Input: part model. Units: mm. Frame: model coordinates. Face numbers are marked on the shaded views. Coordinates: 2 decimals unless noted, no trailing zeros. Loops run counter-clockwise (first coordinate to the right, second up) from the corner with the lowest first, then second, coordinate; pieces in that order, holes last. Notation, with made-up numbers: (15, -22) - (21, -22) arc R23 ccw to (21, -2) - close; hole circle Ø4 at (61, 54.25). An arc over 180 degrees is marked (long way). Write item = value, one per line. Start each with the question number.
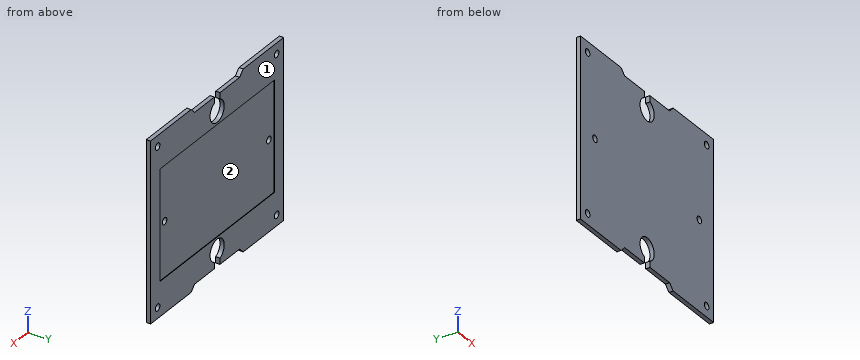
from build123d import *

# Parameters (mm, degrees)
SKETCH1_W              = 94
SKETCH1_H              = 83
SKETCH1_R              = 1.5875
BOSS_EXTRUDE1_DEPTH    = 2
SKETCH2_W              = 81
SKETCH2_H              = 51
CUT_EXTRUDE1_DEPTH     = 0.2
CUT_EXTRUDE2_START     = -2
CUT_EXTRUDE2_OUTLINE_R = 1.6
CUT_EXTRUDE2_DEPTH     = 2


# Read off the part's stored shape, not the designer's step: Cut-Extrude2
with BuildPart() as part:
    # Sketch1 → Boss-Extrude1 (new body)
    with BuildSketch(Plane(origin=(0, 0, 0), x_dir=(1, 0, 0), z_dir=(0, 1, 0))):
        Rectangle(SKETCH1_W, SKETCH1_H)
        with Locations(Location((-42, 36.5, 0), (0, 0, 270))):
            Circle(SKETCH1_R, mode=Mode.SUBTRACT)
        with Locations(Location((42, 36.5, 0), (0, 0, 270))):
            Circle(SKETCH1_R, mode=Mode.SUBTRACT)
        with Locations(Location((42, -36.5, 0), (0, 0, 270))):
            Circle(SKETCH1_R, mode=Mode.SUBTRACT)
        with Locations(Location((-42, -36.5, 0), (0, 0, 270))):
            Circle(SKETCH1_R, mode=Mode.SUBTRACT)
    extrude(amount=BOSS_EXTRUDE1_DEPTH)

    # Sketch2 → Cut-Extrude1 (cut)
    with BuildSketch(Plane(origin=(0, 2, 0), x_dir=(1, 0, 0), z_dir=(0, 1, 0))):
        Rectangle(SKETCH2_W, SKETCH2_H)
    extrude(amount=-CUT_EXTRUDE1_DEPTH, mode=Mode.SUBTRACT)

    # Cut-Extrude2 outline → Cut-Extrude2 (cut)
    with BuildSketch(Plane(origin=(0, 2, 0), x_dir=(1, 0, 0), z_dir=(0, 1, 0)).offset(CUT_EXTRUDE2_START)):
        with Locations((36.83, 0)):
            Circle(CUT_EXTRUDE2_OUTLINE_R)
        with Locations((-36.83, 0)):
            Circle(CUT_EXTRUDE2_OUTLINE_R)
        with BuildLine():
            Line((15.875, -38.96), (2, -38.96))
            Line((2, -38.96), (2, -36.082575695))
            ThreePointArc((2, -36.082575695), (0, -26.5), (-2, -36.082575695))
            Line((-2, -36.082575695), (-2, -38.96))
            Line((-2, -38.96), (-15.875, -38.96))
            Line((-15.875, -38.96), (-18.415, -41.5))
            Line((-18.415, -41.5), (18.415, -41.5))
            Line((18.415, -41.5), (15.875, -38.96))
        make_face()
        with BuildLine():
            Line((2, 36.082575695), (2, 38.96))
            Line((2, 38.96), (15.875, 38.96))
            Line((15.875, 38.96), (18.415, 41.5))
            Line((18.415, 41.5), (-18.415, 41.5))
            Line((-18.415, 41.5), (-15.875, 38.96))
            Line((-15.875, 38.96), (-2, 38.96))
            Line((-2, 38.96), (-2, 36.082575695))
            ThreePointArc((-2, 36.082575695), (0, 26.5), (2, 36.082575695))
        make_face()
    extrude(amount=CUT_EXTRUDE2_DEPTH, mode=Mode.SUBTRACT)


solid = part.part
Item 1: Cut plane C-C on x = 36.83. Return loops of the section in (y, z).
Item 2: Cut plane D-D on z = 7.5. Return loops of the section in (x, y).
Item 3: Pull-direction query (Z, two-part tool) for the marked faces 1 and 2; classes: pulls with the +Z half, pulls with the -Z half, needs draft (parallel to the pull), parting line crosses it, or undercut.
Item 4: Cut plane B-B on z = -31.5. Return loops of the section in (x, y), plus the area to 3 significant figures.
Item 5: Cut plane A-A on y = 1.3. Return loops of the section in (x, z) (1 decimal).
Item 6: Ray query, line 1 (X direction, y = 1, z = 0); line 2 (X direction, y = 1.4, z = -36.5); line 3 (X direction, y = 1, z = -0.5). Return the intervals inside material, ascending.
Item 7: Pin query (flat end, axial travel): pin 1 (5 mm diameter, centred on x = 8, z = -7, fed in from +Y); pin 2 (6 mm diameter, centred on x = 0, z = -31.5, fed in from +Y); pin 3 (1 mm diameter, centred on x = -4.5, y = 1.5, fed in from +Z). Return the tip coordinate at first contact, or that it passes through.
Recorded:
q1.outline = (0, -41.5) - (2, -41.5) - (2, -25.5) - (1.8, -25.5) - (1.8, -1.6) - (0, -1.6) - close; (0, 1.6) - (1.8, 1.6) - (1.8, 25.5) - (2, 25.5) - (2, 41.5) - (0, 41.5) - close
q2.outline = (-47, 0) - (47, 0) - (47, 2) - (40.5, 2) - (40.5, 1.8) - (-40.5, 1.8) - (-40.5, 2) - (-47, 2) - close
q3.face_1 = needs draft
q3.face_2 = undercut
q4.outline = (-47, 0) - (-5, 0) - (-5, 2) - (-47, 2) - close; (5, 0) - (47, 0) - (47, 2) - (5, 2) - close
q4.area = 168 mm²
q5.outline = (-47, -41.5) - (-18.4, -41.5) - (-15.9, -39) - (-2, -39) - (-2, -36.1) arc R5 cw (long way) to (2, -36.1) - (2, -39) - (15.9, -39) - (18.4, -41.5) - (47, -41.5) - (47, 41.5) - (18.4, 41.5) - (15.9, 39) - (2, 39) - (2, 36.1) arc R5 cw (long way) to (-2, 36.1) - (-2, 39) - (-15.9, 39) - (-18.4, 41.5) - (-47, 41.5) - close; hole circle Ø3.2 at (-42, -36.5); hole circle Ø3.2 at (-42, 36.5); hole circle Ø3.2 at (-36.8, 0); hole circle Ø3.2 at (36.8, 0); hole circle Ø3.2 at (42, -36.5); hole circle Ø3.2 at (42, 36.5)
q6.line_1 = -47 to -38.43, -35.23 to 35.23, 38.43 to 47
q6.line_2 = -47 to -43.59, -40.41 to -2, 2 to 40.41, 43.59 to 47
q6.line_3 = -47 to -38.35, -35.31 to 35.31, 38.35 to 47
q7.pin_1 = 1.8
q7.pin_2 = through
q7.pin_3 = 38.96
